Design review of the part built by this model. Coordinates are the model's own, in mm. A direction names the side the tool comes from. Coordinates: 2 decimals unless noted, no trailing zeros. Loops run counter-clockwise (first coordinate to the right, second up) from the corner with the lowest first, then second, coordinate; pieces in that order, holes last. Notation, with made-up numbers: M -13.5,62 L 7.5,62 A18 ccw 7.5,87 Z; hole C -2.5,65 d1. An arc over 180 degrees is marked long. Answer as a JSON object with one key per item and string values. Group by question number.
1. Draft analysis for pull direction Y (two halves, no side actions). For faces 4 (the cylindrical face through (-37.97, -0.62, 3.55)), 5 (the flat face through (-26, 22, 0)), 6 (the flat face through (22.298, 4.997, 3.451)), 7 (the cylindrical face through (-37.844, 42.681, 3.549)), state which applies: +Y half, -Y half, draft (parallel to the pull), parting line (faces both ways), or undercut.
2. Insertion check: pin 1 (1 mm diameter, centred on x = -54.5, z = 2.5, fed in from -Y); pin 2 (3.5 mm diameter, centred on y = 78, z = 2, fed in from -X); pin 3 (2 mm diameter, centred on x = -47, y = -6, fed in from +Z); pin 4 (4 mm diameter, centred on x = 10.5, z = 6, fed in from +Y). Each pin has a flat end and moves straight along its axis. Give the tip position at first contact, or say it passes through.
3. Consider section B-B (y = 62). State the section outline as (x, z) points, then the cut area to 3 significant figures.
4. To check wall thickness, follow probe 1 along X at (y, z) = (63, 2); probe 2 along X at (y, z) = (-18, 5.75); probe 3 along X at (y, z) = (-32, 5.75). State the ranges of each line that lie inside material, in increasing order.
5. Consider section A-A (x = 18.5). State the section outline as (y, z) points.
6. Consider section D-D (y = 84). State the section outline as (x, z) points, then the cut area to 3 significant figures.
7. Consider section C-C (x = -84.5). State the section outline as (y, z) points.
8. Machinability: for faces 1 (the flat face through (-15.408, 70, 3)), 2 (the flat face through (11.74, -12, 3.45)), 3 (the flat face through (-73.113, 36.989, 3.451)), which of the approach directions +Z, -Z, +X, -X, +Y, -Y give a long, thin tool a straight path to every point of the face, cutting with its end or side? Answer none if there is none.
from build123d import *

# Parameters (mm, degrees)
F1_DEPTH = 7
F2_R     = 3
F3_R     = 3
F4_R     = 5


with BuildPart() as f1:
    # F0 (on Top) → F1 (new body)
    with BuildSketch(Plane.XY):
        Polygon((-15.407504, 95.992884), (-35.407504, 95.992884), (-35.407504, 38.313392), (-85.35941, 67.153138), (-95.35941, 49.83263), (-45.407504, 20.992884), (-95.35941, -7.846862), (-85.35941, -25.16737), (-35.407504, 3.672376), (-35.407504, -54.007116), (-15.407504, -54.007116), (-15.407504, 3.672376), (34.544401, -25.16737), (44.544401, -7.846862), (-5.407504, 20.992884), (44.544401, 49.83263), (34.544401, 67.153138), (-15.407504, 38.313392), align=None)
    extrude(amount=F1_DEPTH)

    # F2
    f2_edges = [f1.edges().sort_by_distance(p)[0] for p in [
        (-35.407504, -54.007116, 3.5),
        (-15.407504, -54.007116, 3.5),
        (34.544401, -25.16737, 3.5),
        (44.544401, -7.846862, 3.5),
        (44.544401, 49.83263, 3.5),
        (34.544401, 67.153138, 3.5),
        (-85.35941, -25.16737, 3.5),
        (-95.35941, -7.846862, 3.5),
        (-85.35941, 67.153138, 3.5),
        (-95.35941, 49.83263, 3.5),
        (-35.407504, 95.992884, 3.5),
    ]]
    fillet(f2_edges, radius=F2_R)

    # F3
    f3_edges = [f1.edges().sort_by_distance(p)[0] for p in [
        (-15.407504, 95.992884, 3.5),
    ]]
    fillet(f3_edges, radius=F3_R)

    # F4
    f4_edges = [f1.edges().sort_by_distance(p)[0] for p in [
        (-35.407504, 38.313392, 3.5),
        (-15.407504, 38.313392, 3.5),
        (-5.407504, 20.992884, 3.5),
        (-45.407504, 20.992884, 3.5),
        (-35.407504, 3.672376, 3.5),
        (-15.407504, 3.672376, 3.5),
    ]]
    fillet(f4_edges, radius=F4_R)


solid = f1.part
Findings below:
{
 "1": {"face 4": "-Y half", "face 5": "draft", "face 6": "undercut", "face 7": "+Y half"},
 "2": {"pin 1": "stops at y = -7.64", "pin 2": "stops at x = -35.41", "pin 3": "passes through", "pin 4": "stops at y = 54.43"},
 "3": {"outline": "M -88.33,0 L -76.43,0 L -76.43,7 L -88.33,7 Z; M -35.41,0 L -15.41,0 L -15.41,7 L -35.41,7 Z; M 25.62,0 L 37.52,0 L 37.52,7 L 25.62,7 Z", "area": "307 mm^2"},
 "4": {"probe 1": "x = -87.76 to -78.17, -35.41 to -15.41, 27.35 to 36.94", "probe 2": "x = -89.5 to -72.95, -35.41 to -15.41, 22.13 to 38.68", "probe 3": "x = -35.41 to -15.41"},
 "5": {"outline": "M -15.9,0 L 7.19,0 L 7.19,7 L -15.9,7 Z; M 34.8,0 L 57.89,0 L 57.89,7 L 34.8,7 Z"},
 "6": {"outline": "M -35.41,0 L -15.41,0 L -15.41,7 L -35.41,7 Z", "area": "140 mm^2"},
 "7": {"outline": "M -24.06,0 L -1.58,0 L -1.58,7 L -24.06,7 Z; M 43.56,0 L 66.05,0 L 66.05,7 L 43.56,7 Z"},
 "8": {"face 1": "+Z, -Z, +Y", "face 2": "+Z, -Z, -Y", "face 3": "+Z, -Z, -X"}
}
